from build123d import *

# Parameters (mm, degrees)
F0_W     = 50.8
F0_H     = 76.2
F1_DEPTH = 15.748
F2_R     = 16.174044
F3_DEPTH = 25.4
F4_W     = 25.4
F4_H     = 76.2
F5_DEPTH = 43.18
F6_W     = 25.4
F6_H     = 25.4
F7_DEPTH = 21.59


with BuildPart() as f1:
    # F0 (on Top) → F1 (new body)
    with BuildSketch(Plane.XY):
        Rectangle(F0_W, F0_H)
        with BuildLine():
            Line((-25.4, -38.1), (-25.4, 38.1))
            ThreePointArc((-25.4, 38.1), (-63.5, 0), (-25.4, -38.1))
        make_face()
    extrude(amount=F1_DEPTH)

    # F2 (on face) → F3 (cut)
    with BuildSketch(Plane.XY.offset(15.748)):
        with Locations((-30.42051, 0)):
            Circle(F2_R)
    extrude(amount=-F3_DEPTH, mode=Mode.SUBTRACT)

    # F4 (on face) → F5 (join)
    with BuildSketch(Plane.XY.offset(15.748)):
        with Locations((12.7, 0)):
            Rectangle(F4_W, F4_H)
    extrude(amount=F5_DEPTH)

    # F6 (on face) → F7 (cut)
    with BuildSketch(Plane.XY.offset(58.928)):
        with Locations((12.7, 25.4)):
            Rectangle(F6_W, F6_H)
    extrude(amount=-F7_DEPTH, mode=Mode.SUBTRACT)


solid = f1.part
The model under review builds one solid part; all positions refer to its coordinate system, in mm. A direction names the side the tool comes from. Coordinates: 2 decimals unless noted, no trailing zeros. Loops run counter-clockwise (first coordinate to the right, second up) from the corner with the lowest first, then second, coordinate; pieces in that order, holes last. Notation, with made-up numbers: (-33.75, -1) -> (15.25, -1) arc R19 cw to (15.25, 23) -> close; hole circle Ø7 at (-40, 23). An arc over 180 degrees is marked (long way). Use a Markdown table: item, result. Add a question column.
1. To check wall thickness, follow line 1 (X direction, y = -2, z = 45); line 2 (Z direction, x = -35, y = -16.5); line 3 (Y direction, x = -17.5, z = 6.5). State the ranges of each line that lie inside material, in increasing order.
2. Add section C-C on x = 9. Write out the cut boundary in (y, z).
3. Machinability: for faces 1 (the face through (-10, 1, 0)), 2 (the face through (-25, -16, 15.748)), 3 (the face through (13, 12.7, 48)), which of the approach directions +Z, -Z, +X, -X, +Y, -Y give a long, thin tool a straight path to every point of the face, cutting with its end or side? Answer none if there is none.
4. Add section B-B on z = 7. Write out the cut boundary in (x, y).
5. Clearance check with flat-ended pins moving along their axes: pin 1 Ø21.5 at (y, z) = (11, 44) entering from -X; pin 2 Ø12.5 at (x, y) = (15.5, 20) entering from +Z; pin 3 Ø10 at (x, z) = (-51.5, 9) entering from +Y. State where each tip first meets the part, or that it passes through.
6. Add section D-D on x = -16. Write out the cut boundary in (y, z).
7. Add section A-A on y = 0. Write out the cut boundary in (x, z).
Returned:
| question | item | result |
|---|---|---|
| 1 | line 1 | x = 0 to 25.4 |
| 1 | line 2 | z = 0 to 15.75 |
| 1 | line 3 | y = -38.1 to -9.73, 9.73 to 38.1 |
| 2 | outline | (-38.1, 0) -> (38.1, 0) -> (38.1, 37.34) -> (12.7, 37.34) -> (12.7, 58.93) -> (-38.1, 58.93) -> close |
| 3 | face 1 | -Z, +X, -X, +Y, -Y |
| 3 | face 2 | +Z, -X, +Y, -Y |
| 3 | face 3 | +Z, +X, -X, +Y |
| 4 | outline | (-25.4, -38.1) -> (25.4, -38.1) -> (25.4, 38.1) -> (-25.4, 38.1) arc R38.1 ccw to start; hole circle Ø32.35 at (-30.42, 0) |
| 5 | pin 1 | stops at x = 0 |
| 5 | pin 2 | stops at z = 37.34 |
| 5 | pin 3 | stops at y = 31.72 |
| 6 | outline | (-38.1, 0) -> (-7.32, 0) -> (-7.32, 15.75) -> (-38.1, 15.75) -> close; (7.32, 0) -> (38.1, 0) -> (38.1, 15.75) -> (7.32, 15.75) -> close |
| 7 | outline | (-63.5, 0) -> (-46.59, 0) -> (-46.59, 15.75) -> (-63.5, 15.75) -> close; (-14.25, 0) -> (25.4, 0) -> (25.4, 58.93) -> (0, 58.93) -> (0, 15.75) -> (-14.25, 15.75) -> close |
